Geometry check sheet. Reference: the model listing, model coordinates, mm. A direction names the side the tool comes from. Give positions to 0.01 mm unless a question says otherwise; leave off trailing zeros. Write each loop counter-clockwise with the first axis right and the second up, starting at its lowest first coordinate (ties: lowest second). Pieces come first, ordered by that corner, then holes. Notation, with made-up numbers: M 22,-6.75 L 66,-6.75 A24 ccw 66,5.25 Z; hole C 3.25,69 d11. An arc over 180 degrees is marked long. One line per item, written item: value. Start each with the question number.
1. Gauge pin test, flat ends, axial feed: pin 1 (1.5 mm diameter, centred on y = 7.15, z = 25, fed in from -X); pin 2 (2 mm diameter, centred on y = 22.85, z = 25, fed in from -X); pin 3 (0.6 mm diameter, centred on x = 14, z = 13, fed in from +Y). Record the tip position at first contact, or that the pin passes through.
2. Release check for a two-part mould opening along Z. For faces 1 (the face through (21.13, 21.6, 25.05)), 2 (the face through (14.5, 2, 25)) record: pulls with the +Z half, pulls with the -Z half, needs draft (parallel to the pull), parting line crosses it, or undercut.
3. Tool access check on faces 3 (the face through (19, 5, 25)), 4 (the face through (19.5, 27, 25)), 5 (the face through (27.17, 5.9, 25.05)), 6 (the face through (5, 19, 25)), 7 (the face through (28, 10.5, 25)). Record the directions out of +Z, -Z, +X, -X, +Y, -Y that give a thin tool (end or side, any length) a straight path to the whole face; none if there is none.
4. Scan lines: line 1 (Y direction, x = 25.5, z = 8.5); line 2 (Z direction, x = 22.85, y = 27). Record each from-to range of solid material in increasing order.
5. Cross-section at A-A on y = 9.25. Record the cut outline in (x, z).
from build123d import *

# Parameters (mm, degrees)
SKETCH1_W                        = 30
SKETCH1_H                        = 30
BOSS_EXTRUDE1_DEPTH              = 50
FILLET1_R                        = 1
CUT_EXTRUDE2_START               = -30
CUT_EXTRUDE2_OUTLINE_R           = 6.425
CUT_EXTRUDE2_DEPTH               = 30
TAP_DRILL_FOR_M3_TAP1_D          = 2.5
TAP_DRILL_FOR_M3_TAP2_AT_2_COUNT = 2
TAP_DRILL_FOR_M3_TAP2_AT_2_PITCH = 15.7
CUT_EXTRUDE5_REACH               = 67.574
SKETCH6_W                        = 1.5
SKETCH6_H                        = 5
FILLET2_R                        = 0.2
CIRPATTERN1_DEPTH                = 50
CIRPATTERN1_2_OUTLINE_R          = 1.25
CIRPATTERN1_2_DEPTH              = 7.1500001
CIRPATTERN1_START                = 22.8499999
CIRPATTERN1_3_OUTLINE_R          = 1.25
CIRPATTERN1_3_DEPTH              = 7.1500001


# Read off the part's stored shape, not the designer's step: Cut-Extrude2, CirPattern1
with BuildPart() as part:
    # Sketch1 → Boss-Extrude1 (new body)
    with BuildSketch(Plane.XY):
        with Locations((15, 15)):
            Rectangle(SKETCH1_W, SKETCH1_H)
    extrude(amount=BOSS_EXTRUDE1_DEPTH)

    # Fillet1
    fillet1_edges = [part.edges().sort_by_distance(p)[0] for p in [
        (0, 30, 25),
        (30, 30, 25),
        (30, 0, 25),
        (0, 0, 25),
    ]]
    fillet(fillet1_edges, radius=FILLET1_R)

    # Cut-Extrude2 outline → Cut-Extrude2 (cut)
    with BuildSketch(Plane.XY.offset(50).offset(CUT_EXTRUDE2_START)):
        with Locations((15, 15)):
            Circle(CUT_EXTRUDE2_OUTLINE_R)
    extrude(amount=CUT_EXTRUDE2_DEPTH, mode=Mode.SUBTRACT)

    # Tap Drill for M3 Tap1 (through all)
    with Locations(Plane(origin=(0, 0, 0), x_dir=(-1, 0, 0), z_dir=(0, -1, 0))):
        with Locations((-7.15, -25), (-22.85, -25)):
            Hole(TAP_DRILL_FOR_M3_TAP1_D / 2)

    # Sketch8 → Tap Drill for M3 Tap2 (revolve, cut)
    with BuildSketch(Plane(origin=(7.15, 0, 25), x_dir=(0, 0, -1), z_dir=(1, 0, 0))):
        Polygon((0, 0), (0, 10.751075774), (1.25, 10), (1.25, 0), align=None)
    tap_drill_for_m3_tap2 = revolve(axis=Axis((7.15, -6.35, 25), (0, 1, 0)), mode=Mode.SUBTRACT)

    # Tap Drill for M3 Tap2 at 2: Tap Drill for M3 Tap2 ×2
    with Locations(*[(i * TAP_DRILL_FOR_M3_TAP2_AT_2_PITCH, 0, 0) for i in range(1, TAP_DRILL_FOR_M3_TAP2_AT_2_COUNT)]):
        add(tap_drill_for_m3_tap2, mode=Mode.SUBTRACT)

    # Sketch6 → Cut-Extrude5 (cut, up to next)
    with BuildSketch(Plane.XY.offset(50), mode=Mode.PRIVATE) as cut_extrude5_sk1:
        with Locations((11.25, 27.5)):
            Rectangle(SKETCH6_W, SKETCH6_H)
    cut_extrude5_tool1 = extrude(cut_extrude5_sk1.sketch, amount=-CUT_EXTRUDE5_REACH, mode=Mode.PRIVATE) & part.part
    # Sketch6 → Cut-Extrude5 (cut, up to next)
    with BuildSketch(Plane.XY.offset(50), mode=Mode.PRIVATE) as cut_extrude5_sk2:
        with Locations((18.75, 27.5)):
            Rectangle(SKETCH6_W, SKETCH6_H)
    cut_extrude5_tool2 = extrude(cut_extrude5_sk2.sketch, amount=-CUT_EXTRUDE5_REACH, mode=Mode.PRIVATE) & part.part
    # Sketch6 → Cut-Extrude5 (cut, up to next)
    with BuildSketch(Plane.XY.offset(50), mode=Mode.PRIVATE) as cut_extrude5_sk3:
        with Locations((13.75, 27.5)):
            Rectangle(SKETCH6_W, SKETCH6_H)
    cut_extrude5_tool3 = extrude(cut_extrude5_sk3.sketch, amount=-CUT_EXTRUDE5_REACH, mode=Mode.PRIVATE) & part.part
    # Sketch6 → Cut-Extrude5 (cut, up to next)
    with BuildSketch(Plane.XY.offset(50), mode=Mode.PRIVATE) as cut_extrude5_sk4:
        with Locations((16.25, 27.5)):
            Rectangle(SKETCH6_W, SKETCH6_H)
    cut_extrude5_tool4 = extrude(cut_extrude5_sk4.sketch, amount=-CUT_EXTRUDE5_REACH, mode=Mode.PRIVATE) & part.part
    add(cut_extrude5_tool1.solids().sort_by_distance((11.25, 27.5, 50))[0], mode=Mode.SUBTRACT)
    add(cut_extrude5_tool2.solids().sort_by_distance((18.75, 27.5, 50))[0], mode=Mode.SUBTRACT)
    add(cut_extrude5_tool3.solids().sort_by_distance((13.75, 27.5, 50))[0], mode=Mode.SUBTRACT)
    add(cut_extrude5_tool4.solids().sort_by_distance((16.25, 27.5, 50))[0], mode=Mode.SUBTRACT)

    # Fillet2
    fillet2_edges = [part.edges().sort_by_distance(p)[0] for p in [
        (18, 25, 25),
        (18, 30, 25),
        (19.5, 30, 25),
        (19.5, 25, 25),
        (10.5, 30, 25),
        (12, 30, 25),
        (12, 25, 25),
        (10.5, 25, 25),
        (13, 30, 25),
        (14.5, 30, 25),
        (14.5, 25, 25),
        (13, 25, 25),
        (15.5, 30, 25),
        (17, 30, 25),
        (17, 25, 25),
        (15.5, 25, 25),
    ]]
    fillet(fillet2_edges, radius=FILLET2_R)

    # CirPattern1 outline → CirPattern1 (cut)
    with BuildSketch(Plane.XY):
        with BuildLine():
            Line((10.5, 0), (12, 0))
            Line((12, 0), (12, 4.8))
            ThreePointArc((12, 4.8), (11.941421356, 4.941421356), (11.8, 5))
            Line((11.8, 5), (10.7, 5))
            ThreePointArc((10.7, 5), (10.558578644, 4.941421356), (10.5, 4.8))
            Line((10.5, 4.8), (10.5, 0))
        make_face()
        with BuildLine():
            Line((18, 4.8), (18, 0))
            Line((18, 0), (19.5, 0))
            Line((19.5, 0), (19.5, 4.8))
            ThreePointArc((19.5, 4.8), (19.441421356, 4.941421356), (19.3, 5))
            Line((19.3, 5), (18.2, 5))
            ThreePointArc((18.2, 5), (18.058578644, 4.941421356), (18, 4.8))
        make_face()
        with BuildLine():
            Line((15.5, 4.8), (15.5, 0))
            Line((15.5, 0), (17, 0))
            Line((17, 0), (17, 4.8))
            ThreePointArc((17, 4.8), (16.941421356, 4.941421356), (16.8, 5))
            Line((16.8, 5), (15.7, 5))
            ThreePointArc((15.7, 5), (15.558578644, 4.941421356), (15.5, 4.8))
        make_face()
        with BuildLine():
            Line((13, 4.8), (13, 0))
            Line((13, 0), (14.5, 0))
            Line((14.5, 0), (14.5, 4.8))
            ThreePointArc((14.5, 4.8), (14.441421356, 4.941421356), (14.3, 5))
            Line((14.3, 5), (13.2, 5))
            ThreePointArc((13.2, 5), (13.058578644, 4.941421356), (13, 4.8))
        make_face()
        with BuildLine():
            ThreePointArc((5, 11.8), (4.941421356, 11.941421356), (4.8, 12))
            Line((4.8, 12), (0, 12))
            Line((0, 12), (0, 10.5))
            Line((0, 10.5), (4.8, 10.5))
            ThreePointArc((4.8, 10.5), (4.941421356, 10.558578644), (5, 10.7))
            Line((5, 10.7), (5, 11.8))
        make_face()
        with BuildLine():
            Line((0, 19.5), (0, 18))
            Line((0, 18), (4.8, 18))
            ThreePointArc((4.8, 18), (4.941421356, 18.058578644), (5, 18.2))
            Line((5, 18.2), (5, 19.3))
            ThreePointArc((5, 19.3), (4.941421356, 19.441421356), (4.8, 19.5))
            Line((4.8, 19.5), (0, 19.5))
        make_face()
        with BuildLine():
            Line((0, 17), (0, 15.5))
            Line((0, 15.5), (4.8, 15.5))
            ThreePointArc((4.8, 15.5), (4.941421356, 15.558578644), (5, 15.7))
            Line((5, 15.7), (5, 16.8))
            ThreePointArc((5, 16.8), (4.941421356, 16.941421356), (4.8, 17))
            Line((4.8, 17), (0, 17))
        make_face()
        with BuildLine():
            Line((0, 14.5), (0, 13))
            Line((0, 13), (4.8, 13))
            ThreePointArc((4.8, 13), (4.941421356, 13.058578644), (5, 13.2))
            Line((5, 13.2), (5, 14.3))
            ThreePointArc((5, 14.3), (4.941421356, 14.441421356), (4.8, 14.5))
            Line((4.8, 14.5), (0, 14.5))
        make_face()
        with BuildLine():
            Line((30, 10.5), (30, 12))
            Line((30, 12), (25.2, 12))
            ThreePointArc((25.2, 12), (25.058578644, 11.941421356), (25, 11.8))
            Line((25, 11.8), (25, 10.7))
            ThreePointArc((25, 10.7), (25.058578644, 10.558578644), (25.2, 10.5))
            Line((25.2, 10.5), (30, 10.5))
        make_face()
        with BuildLine():
            Line((25.2, 18), (30, 18))
            Line((30, 18), (30, 19.5))
            Line((30, 19.5), (25.2, 19.5))
            ThreePointArc((25.2, 19.5), (25.058578644, 19.441421356), (25, 19.3))
            Line((25, 19.3), (25, 18.2))
            ThreePointArc((25, 18.2), (25.058578644, 18.058578644), (25.2, 18))
        make_face()
        with BuildLine():
            Line((25.2, 15.5), (30, 15.5))
            Line((30, 15.5), (30, 17))
            Line((30, 17), (25.2, 17))
            ThreePointArc((25.2, 17), (25.058578644, 16.941421356), (25, 16.8))
            Line((25, 16.8), (25, 15.7))
            ThreePointArc((25, 15.7), (25.058578644, 15.558578644), (25.2, 15.5))
        make_face()
        with BuildLine():
            Line((25.2, 13), (30, 13))
            Line((30, 13), (30, 14.5))
            Line((30, 14.5), (25.2, 14.5))
            ThreePointArc((25.2, 14.5), (25.058578644, 14.441421356), (25, 14.3))
            Line((25, 14.3), (25, 13.2))
            ThreePointArc((25, 13.2), (25.058578644, 13.058578644), (25.2, 13))
        make_face()
    extrude(amount=CIRPATTERN1_DEPTH, mode=Mode.SUBTRACT)

    # CirPattern1 2 outline → CirPattern1 2 (cut)
    with BuildSketch(Plane.YZ):
        with Locations((22.85, 25)):
            Circle(CIRPATTERN1_2_OUTLINE_R)
        with Locations((7.15, 25)):
            Circle(CIRPATTERN1_2_OUTLINE_R)
    extrude(amount=CIRPATTERN1_2_DEPTH, mode=Mode.SUBTRACT)

    # CirPattern1 3 outline → CirPattern1 3 (cut)
    with BuildSketch(Plane.YZ.offset(CIRPATTERN1_START)):
        with Locations((22.85, 25)):
            Circle(CIRPATTERN1_3_OUTLINE_R)
        with Locations((7.15, 25)):
            Circle(CIRPATTERN1_3_OUTLINE_R)
    extrude(amount=CIRPATTERN1_3_DEPTH, mode=Mode.SUBTRACT)

    # CirPattern1 4 outline → CirPattern1 4 (revolve, cut)
    with BuildSketch(Plane(origin=(0, 22.85, 25), x_dir=(0, 1, 0), z_dir=(0, 0, -1))):
        Polygon((0, 19.248924226), (1.25, 20), (1.25, 22.85), (0, 22.85), align=None)
        Polygon((1.25, 10), (0, 10.751075774), (0, 7.15), (1.25, 7.15), align=None)
    revolve(axis=Axis((0, 22.85, 25), (1, 0, 0)), mode=Mode.SUBTRACT)

    # CirPattern1 5 outline → CirPattern1 5 (revolve, cut)
    with BuildSketch(Plane(origin=(0, 7.15, 25), x_dir=(0, 1, 0), z_dir=(0, 0, -1))):
        Polygon((0, 19.248924226), (1.25, 20), (1.25, 22.85), (0, 22.85), align=None)
        Polygon((1.25, 10), (0, 10.751075774), (0, 7.15), (1.25, 7.15), align=None)
    revolve(axis=Axis((0, 7.15, 25), (1, 0, 0)), mode=Mode.SUBTRACT)


solid = part.part
Report:
1. pin 1: stops at x = 10.3
1. pin 2: stops at x = 10.15
1. pin 3: stops at y = 25
2. face 1: undercut
2. face 2: needs draft
3. face 3: +Z, -Z, -Y
3. face 4: +Z, -Z, +Y
3. face 5: +X
3. face 6: +Z, -Z, -X
3. face 7: +Z, -Z, +X
4. line 1: y = 0 to 10.5, 12 to 13, 14.5 to 15.5, 17 to 18, 19.5 to 30
4. line 2: z = 0 to 23.75, 26.25 to 50
5. outline: M 0,0 L 30,0 L 30,50 L 17.87,50 L 17.87,20 L 12.13,20 L 12.13,50 L 0,50 Z; hole C 7.15,25 d2.5; hole C 22.85,25 d2.5
